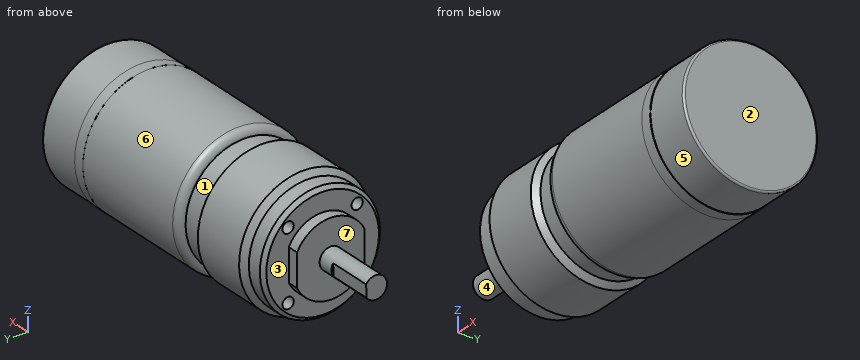
```python
from build123d import *

# Parameters (mm, degrees)
SKETCH_1_W               = 16.3
SKETCH_1_H               = 3
SKETCH_1_W_2             = 5
SKETCH_1_H_2             = 16
SKETCH_4_R               = 18
EXTRUDE_1_DEPTH          = 14
SKETCH_5_R               = 18
CUT_EXTRUDE_2_DEPTH      = 3.5
CUT_EXTRUDE_4_DEPTH      = 12
SKETCH_8_W               = 12
SKETCH_8_H               = 0.1
FILLET_3_R               = 0.5
SKETCH_10_W              = 3
SKETCH_10_H              = 0.01
CUT_EXTRUDE_6_DEPTH      = 3
SKETCH_13_R              = 1.5
CUT_EXTRUDE_8_DEPTH      = 7
PATTERN_CIRCULAR_2_COUNT = 4


with BuildPart() as part:
    # Эскиз1 → Повернуть1 (revolve)
    with BuildSketch(Plane(origin=(0, 0, 0), x_dir=(1, 0, 0), z_dir=(0, 1, 0))):
        with Locations((8.15, 1.5)):
            Rectangle(SKETCH_1_W, SKETCH_1_H)
        Polygon((16.3, 0), (19.3, 0), (19.3, 10), (16.3, 10), (16.3, 3), align=None)
        Polygon((24.3, 0), (24.3, 16), (20.3, 16), (19.3, 15), (19.3, 10), (19.3, 0), align=None)
        Polygon((40.8, 17.5), (42.3, 16), (42.3, 0), (24.3, 0), (24.3, 16), (25.8, 17.5), align=None)
        with Locations((44.8, 8)):
            Rectangle(SKETCH_1_W_2, SKETCH_1_H_2)
        with BuildLine():
            ThreePointArc((47.3, 16), (47.885786438, 17.414213562), (49.3, 18))
            Line((49.3, 18), (86.4, 18))
            Line((86.4, 18), (86.4, 0))
            Line((86.4, 0), (47.3, 0))
            Line((47.3, 0), (47.3, 16))
        make_face()
    revolve(axis=Axis((0, 0, 0), (1, 0, 0)))

    # Эскиз4 → Бобышка-Вытянуть1 (add)
    with BuildSketch(Plane(origin=(86.4, 0, 0), x_dir=(0, 0, -1), z_dir=(1, 0, 0))):
        Circle(SKETCH_4_R)
    extrude(amount=EXTRUDE_1_DEPTH)

    # Эскиз5 → Вырез-Вытянуть2 (cut)
    with BuildSketch(Plane(origin=(100.4, 0, 0), x_dir=(0, 0, -1), z_dir=(1, 0, 0))):
        Circle(SKETCH_5_R)
    extrude(amount=-CUT_EXTRUDE_2_DEPTH, mode=Mode.SUBTRACT)

    # Эскиз6 → Вырез-Вытянуть4 (cut)
    with BuildSketch(Plane.ZY):
        with BuildLine():
            Line((-1.75306936, 2.434491286), (1.561110291, 2.561822527))
            ThreePointArc((1.561110291, 2.561822527), (-0.115175441, 2.997788288), (-1.75306936, 2.434491286))
        make_face()
    extrude(amount=-CUT_EXTRUDE_4_DEPTH, mode=Mode.SUBTRACT)

    # Вырез-По траектории3: sweep along a path in Эскиз9
    with BuildLine(Plane(origin=(96.9, 0, 0), x_dir=(0, 0, -1), z_dir=(1, 0, 0))) as sweep_3_path:
        CenterArc((0, 0), 17.9, 0, 360)
    # Эскиз8 → Вырез-По траектории3 (sweep, cut)
    with BuildSketch(Plane(origin=(0, 0, 0), x_dir=(1, 0, 0), z_dir=(0, 1, 0))):
        with Locations((90.9, -17.95)):
            Rectangle(SKETCH_8_W, SKETCH_8_H)
    sweep(path=sweep_3_path.line, mode=Mode.SUBTRACT)

    # Скругление3
    fillet_3_edges = [part.edges().sort_by_distance(p)[0] for p in [
        (96.9, 0, 17.9),
    ]]
    fillet(fillet_3_edges, radius=FILLET_3_R)

    # Эскиз10 → Повернуть2 (revolve)
    with BuildSketch(Plane(origin=(0, 0, 0), x_dir=(1, 0, 0), z_dir=(0, 1, 0))):
        with Locations((83.4, 18.005)):
            Rectangle(SKETCH_10_W, SKETCH_10_H)
    revolve(axis=Axis((0, 0, 0), (1, 0, 0)))

    # Эскиз11 → Вырез-Вытянуть6 (cut)
    with BuildSketch(Plane.ZY.offset(-16.3)):
        with BuildLine():
            ThreePointArc((4.358898944, 9), (0, 10), (-4.358898944, 9))
            Line((-4.358898944, 9), (4.358898944, 9))
        make_face()
        with BuildLine():
            Line((4.358898944, -9), (-4.358898944, -9))
            ThreePointArc((-4.358898944, -9), (0, -10), (4.358898944, -9))
        make_face()
    extrude(amount=-CUT_EXTRUDE_6_DEPTH, mode=Mode.SUBTRACT)

    # Эскиз13 → Вырез-Вытянуть8 (cut)
    with BuildSketch(Plane.ZY.offset(-19.3)):
        with Locations((-9.192388155, 9.192388155)):
            Circle(SKETCH_13_R)
    cut_extrude_8 = extrude(amount=-CUT_EXTRUDE_8_DEPTH, mode=Mode.SUBTRACT)

    # Круговой массив2: Вырез-Вытянуть8 ×4 about axis
    pattern_circular_2_axis = Axis((0, 0, 0), (1, 0, 0))
    for i in range(1, PATTERN_CIRCULAR_2_COUNT):
        add(cut_extrude_8.rotate(pattern_circular_2_axis, i * 360 / PATTERN_CIRCULAR_2_COUNT), mode=Mode.SUBTRACT)


solid = part.part
```
Source: CAD feature listing. Evaluate the final solid. Frame: model axes, mm. Face numbers are marked on the shaded views. A direction names the side the tool comes from. Round coordinates to 2 decimals unless told otherwise and drop trailing zeros. Loops run counter-clockwise (first coordinate to the right, second up) from the corner with the lowest first, then second, coordinate; pieces in that order, holes last. Notation, with made-up numbers: M 71.5,63.5 L 91.5,63.5 A13 cw 91.5,77.5 Z; hole C -40,-7 d9. An arc over 180 degrees is marked long. Use a Markdown table: item, result. Add a question column.
1. Cut plane B-B, the plane x = 71.5. Output: boundary loops of the cut face in (y, z).
2. Ray query, line 1 along X through (y, z) = (5.5, -11); line 2 along X through (y, z) = (-9.5, 13.5); line 3 along X through (y, z) = (-3, 1). Return the intervals inside material, ascending. Write a range as [from, to].
3. Cut plane A-A, the plane x = 22. Output: boundary loops of the cut face in (y, z).
4. Contact query for flat-ended pins moving along their axis: pin 1 (8 mm diameter, centred on x = 18, z = 1, fed in from -Y); pin 2 (1.5 mm diameter, centred on x = 40.5, y = 12, fed in from +Z); pin 3 (0.6 mm diameter, centred on y = 3, z = 0.5, fed in from -X); pin 4 (20 mm diameter, centred on y = -3.5, z = -2.5, fed in from -X). Output: stop coordinate, or through.
5. Pull-direction query (X, two-part tool) for the marked faces 1, 2, 3 and 4; classes: +X half, -X half, draft (parallel to the pull), parting line (faces both ways), or undercut.
6. Set-up query: the marked faces 5, 6 and 7. Return all of +Z, -Z, +X, -X, +Y, -Y with unobstructed straight access to the full face (end or side cutting, diameter ignored); none if empty.
Solution:
| question | item | result |
|---|---|---|
| 1 | outline | C 0,0 d36 |
| 2 | line 1 | x = [19.3, 96.9] |
| 2 | line 2 | x = [24.81, 41.79], [47.37, 96.9] |
| 2 | line 3 | x = [16.3, 96.9] |
| 3 | outline | C 0,0 d32; hole C -9.19,-9.19 d3; hole C -9.19,9.19 d3; hole C 9.19,-9.19 d3; hole C 9.19,9.19 d3 |
| 4 | pin 1 | stops at y = -16 |
| 4 | pin 2 | stops at z = 13.4 |
| 4 | pin 3 | stops at x = 12 |
| 4 | pin 4 | stops at x = 0 |
| 5 | face 1 | undercut |
| 5 | face 2 | +X half |
| 5 | face 3 | -X half |
| 5 | face 4 | draft |
| 6 | face 5 | +X |
| 6 | face 6 | +X, -X |
| 6 | face 7 | -X |
